The listing builds one solid part. Answer for the finished solid, in the listing's coordinates (mm). A direction names the side the tool comes from. Coordinates: 2 decimals unless noted, no trailing zeros. Write each loop counter-clockwise with the first axis right and the second up, starting at its lowest first coordinate (ties: lowest second). Pieces come first, ordered by that corner, then holes.
from build123d import *

# Parameters (mm, degrees)
F0_W     = 18.5
F0_H     = 5
F0_W_2   = 3
F0_H_2   = 0.95
F1_DEPTH = 10
F3_DEPTH = 7
F5_DEPTH = 15
F7_DEPTH = 25


with BuildPart() as f1:
    # F0 (on Top) → F1 (new body)
    with BuildSketch(Plane.XY):
        with Locations((4.286429, 2.5)):
            Rectangle(F0_W, F0_H)
        Polygon((-4.963571, 12.05), (-4.963571, 5), (13.536429, 5), (13.536429, 12.05), (10.536429, 12.05), (10.536429, 13), (-1.963571, 13), (-1.963571, 12.05), align=None)
        with Locations((-3.463571, 12.525)):
            Rectangle(F0_W_2, F0_H_2)
        with Locations((12.036429, 12.525)):
            Rectangle(F0_W_2, F0_H_2)
    extrude(amount=F1_DEPTH)

    # F2 (on face) → F3 (cut)
    with BuildSketch(Plane.XZ):
        Polygon((3.859359, 10), (1.959359, 10), (1.959359, 9), (2.959359, 9), (2.959359, 8), (1.959359, 8), (1.959359, 7), (2.959359, 7), (2.959359, 6), (1.959359, 6), (1.959359, 5), (2.959359, 5), (2.959359, 4), (1.959359, 4), (1.959359, 3), (2.959359, 3), (2.959359, 2), (1.959359, 2), (1.959359, 1), (2.959359, 1), (2.959359, 0), (3.859359, 0), align=None)
    extrude(amount=-F3_DEPTH, mode=Mode.SUBTRACT)

    # F4 (on face) → F5 (join)
    with BuildSketch(Plane.XY.offset(10)):
        Polygon((-4.963571, 13), (-4.963571, 7), (1.959359, 7), (3.859359, 7), (13.536429, 7), (13.536429, 13), align=None)
    extrude(amount=F5_DEPTH)

    # F6 (on face) → F7 (cut)
    with BuildSketch(Plane.XZ.offset(-7)):
        with BuildLine():
            Line((6.686429, 13.4), (6.686429, 20.4))
            ThreePointArc((6.686429, 20.4), (5.983486, 22.097056), (4.286429, 22.8))
            ThreePointArc((4.286429, 22.8), (2.589373, 22.097056), (1.886429, 20.4))
            Line((1.886429, 20.4), (1.886429, 13.4))
            ThreePointArc((1.886429, 13.4), (2.589373, 11.702944), (4.286429, 11))
            ThreePointArc((4.286429, 11), (5.983486, 11.702944), (6.686429, 13.4))
        make_face()
    extrude(amount=-F7_DEPTH, mode=Mode.SUBTRACT)


solid = f1.part
Q1. Determine the mould class of faces 4 (the face through (2.5, 3.5, 4)), 5 (the face through (-4.964, 8, 10)), 6 (the face through (1.886, 10, 17)), 7 (the face through (-2, 4, 10)) for opening direction Z: released by +Z, released by -Z, zero draft, split by the parting line, or undercut.
Answers below:
face 4: undercut
face 5: zero draft
face 6: undercut
face 7: released by +Z
Q2. The part is cut by section C-C, the plane y = 8. Write down the section's boundary in (x, z).
Answers below:
outline: (-4.96, 0) - (13.54, 0) - (13.54, 25) - (-4.96, 25) - close; hole (1.89, 13.4) arc R2.4 ccw to (4.29, 11) arc R2.4 ccw to (6.69, 13.4) - (6.69, 20.4) arc R2.4 ccw to (4.29, 22.8) arc R2.4 ccw to (1.89, 20.4) - close
Q3. The part is cut by section D-D, the plane x = 5.25. Write down the section's boundary in (y, z), then the cut area to 3 significant figures.
Answers below:
outline: (0, 0) - (13, 0) - (13, 11.2) - (7, 11.2) - (7, 10) - (0, 10) - close; (7, 22.6) - (13, 22.6) - (13, 25) - (7, 25) - close
area: 152 mm2
Q4. Which of the six approach directions +Z, -Z, +X, -X, +Y, -Y give full straight-line access (tool end or side, diameter ignored) to faces 1 (the face through (2.959, 3.5, 6.5)), 2 (the face through (2.5, 3.5, 7)), 3 (the face through (6.686, 10, 17))?
Answers below:
face 1: +Z, -Z, -Y
face 2: -Y
face 3: +Y, -Y
Q5. The part is cut by section B-B, the plane z = 18.5. Write down the section's boundary in (x, y), then the cut area to 3 significant figures.
Answers below:
outline: (-4.96, 7) - (1.89, 7) - (1.89, 13) - (-4.96, 13) - close; (6.69, 7) - (13.54, 7) - (13.54, 13) - (6.69, 13) - close
area: 82.2 mm2
Q6. The part is cut by section A-A, the plane y = 6.5. Write down the section's boundary in (x, z).
Answers below:
outline: (-4.96, 0) - (2.96, 0) - (2.96, 1) - (1.96, 1) - (1.96, 2) - (2.96, 2) - (2.96, 3) - (1.96, 3) - (1.96, 4) - (2.96, 4) - (2.96, 5) - (1.96, 5) - (1.96, 6) - (2.96, 6) - (2.96, 7) - (1.96, 7) - (1.96, 8) - (2.96, 8) - (2.96, 9) - (1.96, 9) - (1.96, 10) - (-4.96, 10) - close; (3.86, 0) - (13.54, 0) - (13.54, 10) - (3.86, 10) - close
Q7. Find the intervals of material crossed by probe 1 along Z at (x, y) = (2, 6.75); probe 2 along X at (y, z) = (12, 20.5); probe 3 along Y at (x, z) = (11.5, 10.75), in increasing order.
Answers below:
probe 1: z = 0 to 1, 2 to 3, 4 to 5, 6 to 7, 8 to 9
probe 2: x = -4.96 to 1.89, 6.68 to 13.54
probe 3: y = 7 to 13
Q8. Given pin 1 (5 mm diameter, centred on x = 2, y = 3.5, fed in from +Z); pin 2 (0.8 mm diameter, centred on x = 2.5, y = 4.5, fed in from +Z), each flat-ended and moving along its own axis, determine where each tip first touches the part or whether it passes through.
Answers below:
pin 1: stops at z = 10
pin 2: stops at z = 9
